Source: CAD feature listing. Evaluate the final solid. Frame: model axes, mm. A direction names the side the tool comes from. Round coordinates to 2 decimals unless told otherwise and drop trailing zeros. Order: outer loops, then holes, each group sorted by start corner. A loop starts at its lowest first (then second) coordinate and runs counter-clockwise, first axis right, second up. Notation, with made-up numbers: (-13.5, -39.75) -> (35.5, -39.75) arc R35 cw to (35.5, -7.75) -> close; hole circle Ø9 at (5, -8). An arc over 180 degrees is marked (long way). Answer as CSV lines item,"result".
from build123d import *

# Parameters (mm, degrees)
BOSS_EXTRUDE5_DEPTH = 10
FILLET1_R           = 3


with BuildPart() as part:
    # Sketch7 → Boss-Extrude5 (new body)
    with BuildSketch(Plane(origin=(0, 0, 0), x_dir=(0, 0, -1), z_dir=(1, 0, 0))):
        Polygon((0, 0), (0, 5), (-5, 5), (-5, 60), (0, 60), (0, 65), (8, 65), (80, 20), (80, 0), align=None)
    extrude(amount=BOSS_EXTRUDE5_DEPTH)

    # Fillet1
    fillet1_edges = [part.edges().sort_by_distance(p)[0] for p in [
        (0, 65, -4),
        (0, 42.5, -44),
        (0, 10, -80),
        (0, 0, -40),
        (10, 42.5, -44),
        (5, 65, -8),
        (5, 20, -80),
        (5, 0, -80),
        (10, 65, -4),
        (10, 0, -40),
        (10, 10, -80),
    ]]
    fillet(fillet1_edges, radius=FILLET1_R)


solid = part.part
1. Reachability of faces 1 (the flat face through (0, 26, -27)), 2 (the flat face through (5, 62, 0)), 3 (the flat face through (5, 2, 0)) from +Z, -Z, +X, -X, +Y, -Y: full face, straight path, thin tool, end or side. Return the list, or none.
Results below:
face 1,"+Z, -Z, -X, +Y, -Y"
face 2,"+Z, +X, -X, +Y"
face 3,"+Z, +X, -X, -Y"
2. Pin query (flat end, axial travel): pin 1 (1.5 mm diameter, centred on x = 6.5, y = 63, fed in from +Z); pin 2 (2.5 mm diameter, centred on x = 4, z = 1.5, fed in from -Y); pin 3 (4 mm diameter, centred on x = 6.5, z = 3.5, fed in from +Y). Return the tip coordinate at first contact, or that it passes through.
Results below:
pin 1,"z = 0"
pin 2,"y = 5"
pin 3,"y = 60"
3. Line query: L1, parallel to Y at x = 0.5, z = -35.5; L2, parallel to Z at x = 7.25, y = 19.5; L3, parallel to Z at x = 9.25, y = 25. Output: solid intervals per line, ascending. Write a range as [from, to].
Results below:
L1,"[1.34, 46.23]"
L2,"[-79.75, 5]"
L3,"[-70.08, 5]"
4. Section query A-A on x = 5.25. Return loops of the section in (y, z), and give its area (3 significant figures).
Results below:
outline,"(0, -77) arc R3 ccw to (3, -80) -> (18.34, -80) arc R3 ccw to (20.88, -78.59) -> (64.54, -8.73) arc R3 ccw to (65, -7.14) -> (65, 0) -> (60, 0) -> (60, 5) -> (5, 5) -> (5, 0) -> (0, 0) -> close"
area,"3,850 mm2"
